Print and shaded views of the part. All mm, measured from the part's lowest x, y and z. A direction names the side the tool comes from. Coordinates: 2 decimals unless noted, no trailing zeros. Loops run counter-clockwise (first coordinate to the right, second up) from the corner with the lowest first, then second, coordinate; pieces in that order, holes last.
1) Saw through at D-D, the plane z = 14.5. Write the cut outline in (x, y), and give its area (3 significant figures).
2) Saw through at A-A, the plane y = 1.5. Write the cut outline in (x, z), and give its area (3 significant figures).
3) Wall check: line 1 along Z through (x, y) = (13.75, 1.95); line 2 along Z through (x, y) = (3, 2.5); line 3 along Y through (x, z) = (17.25, 16.75). Give the ranges that are in metal, low to high.
4) Pin check, flat tips, straight feed: pin 1 Ø1 at (x, z) = (15, 3) entering from +Y; pin 2 Ø0.8 at (x, y) = (12, 1.5) entering from -Z. Stop position of each tip, or through.
5) Which spindle directions (+Z, -Z, +X, -X, +Y, -Y) get a long thin tool onto all of the face, cutting with end or side? Do the marked faces 1 and 2. Say none if no direction does.
6) Saw through at C-C, the plane z = 7.75. Write the cut outline in (x, y), and give its area (3 significant figures).
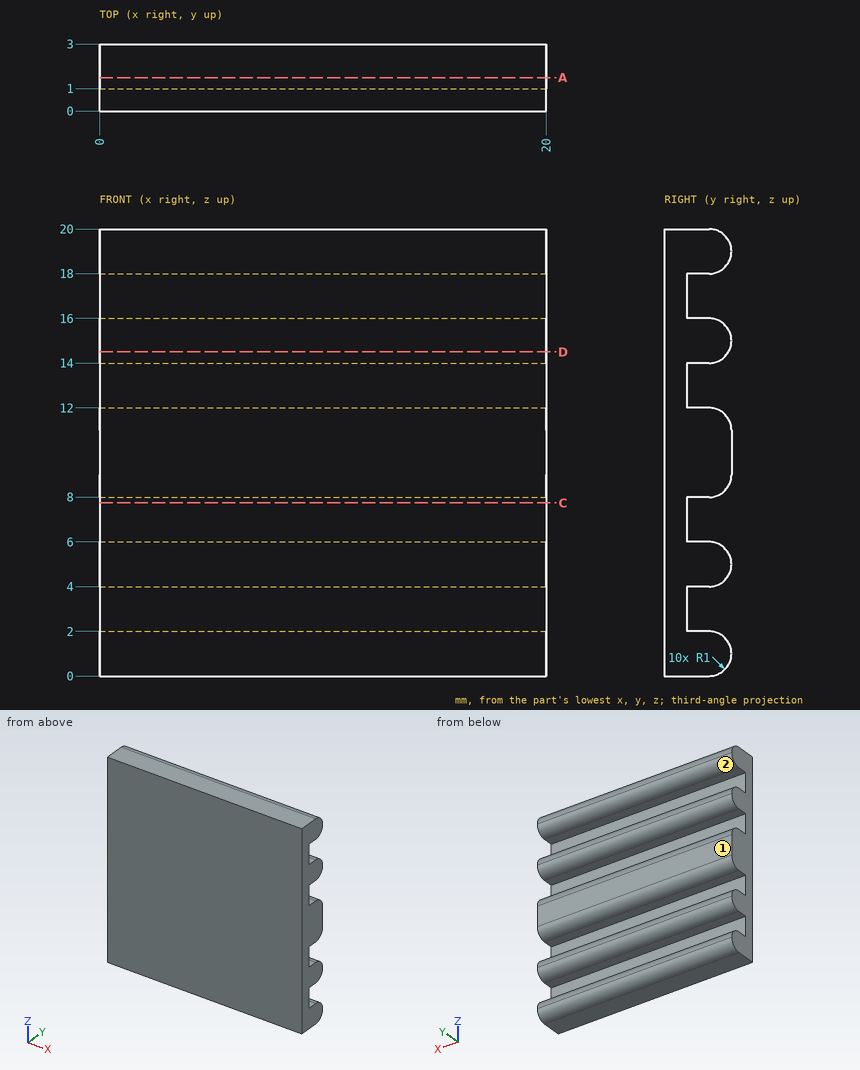
Data:
1. outline: (0, 0) - (20, 0) - (20, 2.87) - (0, 2.87) - close
1. area: 57.3 mm2
2. outline: (0, 0) - (20, 0) - (20, 2) - (0, 2) - close; (0, 4) - (20, 4) - (20, 6) - (0, 6) - close; (0, 8) - (20, 8) - (20, 12) - (0, 12) - close; (0, 14) - (20, 14) - (20, 16) - (0, 16) - close; (0, 18) - (20, 18) - (20, 20) - (0, 20) - close
2. area: 240 mm2
3. line 1: z = 0 to 2, 4 to 6, 8 to 12, 14 to 16, 18 to 20
3. line 2: z = 0.13 to 1.87, 4.13 to 5.87, 8.13 to 11.87, 14.13 to 15.87, 18.13 to 19.87
3. line 3: y = 0 to 1
4. pin 1: stops at y = 1
4. pin 2: stops at z = 0
5. face 1: +Z, -Z, +X, -X, +Y
5. face 2: +X, -X, +Y
6. outline: (0, 0) - (20, 0) - (20, 1) - (0, 1) - close
6. area: 20.0 mm2
